The model under review builds one solid part; all positions refer to its coordinate system, in mm. A direction names the side the tool comes from. Round coordinates to 2 decimals unless told otherwise and drop trailing zeros. Loops run counter-clockwise (first coordinate to the right, second up) from the corner with the lowest first, then second, coordinate; pieces in that order, holes last. Notation, with made-up numbers: M 88.5,-32 L 116.5,-32 A8 cw 116.5,-24 Z; hole C 4,77.25 d3. An arc over 180 degrees is marked long. Return JSON: item names as keys, results as strings. Group by question number.
Q1. Draft analysis for pull direction Y (two halves, no side actions). For faces 5 (the face through (-47.94, 73.48, -0.18)), 6 (the face through (78.134, 0.474, 54.108)), 7 (the face through (89, -11, 44.45)), state which applies: pulls with the +Y half, pulls with the -Y half, needs draft (parallel to the pull), parting line crosses it, or undercut.
Q2. For faces 1 (the face through (63, 0, 57.15)), 2 (the face through (63, 0, 50.8)), 3 (the face through (49.2, -9.6, 52.6)), 4 (the face through (6, 6.35, 33)), list the 3-axis set-ups (+Z, -Z, +X, -X, +Y, -Y) from which the entire face can be reached by the end or side of a thin tool; tool diameter is ignored.
Q3. Consider section A-A (x = -31.75). Count the separate pieces of the cut face and the enclosed holes in it, and give its area (3 significant figures).
Q4. Clearance check with flat-ended pins moving along their axes: pin 1 Ø7 at (y, z) = (8.5, 27) entering from -X; pin 2 Ø24.5 at (x, z) = (52, 31.5) entering from -Y; pin 3 Ø16.5 at (x, y) = (31.75, 53.975) entering from -Z; pin 4 Ø8 at (x, y) = (22.5, -10.5) entering from +Z. State where each tip first meets the part, or that it passes through.
Q5. Consider section B-B (y = 39.5). State the section outline as (x, z) points.
Q6. To check wall thickness, follow line 1 along Y through (x, z) = (31, 7); line 2 along Y through (x, z) = (31.75, 6) (3 decimals); line 3 along Y through (x, z) = (88, 54). State the ranges of each line that lie inside material, in increasing order.
from build123d import *

# Parameters (mm, degrees)
F1_DEPTH = 76.2
F2_DEPTH = 12.7
F3_DEPTH = 6.35
F5_R     = 9.525
F6_R     = 10.7761659596
F7_DEPTH = 76.201
F8_R     = 6.35
F9_DEPTH = 12.7


with BuildPart() as f1:
    # F0 (on Front) → F1 (new body, symmetric)
    with BuildSketch(Plane.XZ):
        Polygon((-50.8, 12.7), (-50.8, -12.7), (50.8, -12.7), (50.8, 12.7), (44.45, 12.7), align=None)
    extrude(amount=F1_DEPTH, both=True)

    # F0 (on Front) → F2 (join, symmetric)
    with BuildSketch(Plane.XZ):
        with BuildLine():
            Line((44.45, 12.7), (50.8, 12.7))
            Line((50.8, 12.7), (50.8, 41.275))
            ThreePointArc((50.8, 41.275), (53.5898079092, 48.0101920908), (60.325, 50.8))
            Line((60.325, 50.8), (88.9, 50.8))
            Line((88.9, 50.8), (88.9, 57.15))
            Line((88.9, 57.15), (60.325, 57.15))
            ThreePointArc((60.325, 57.15), (49.0996798487, 52.5003201513), (44.45, 41.275))
            Line((44.45, 41.275), (44.45, 12.7))
        make_face()
    extrude(amount=F2_DEPTH, both=True)

    # F0 (on Front) → F3 (join, symmetric)
    with BuildSketch(Plane.XZ):
        with BuildLine():
            add(Edge.make_bspline(
                [(-50.8, 12.7), (-36.4359264535, 24.9142696717), (-6.0956798741, 63.0964294524), (39.4712934893, 57.15), (60.325, 57.15)],
                knots=[0, 0, 0, 0, 0.4989893673, 1, 1, 1, 1], degree=3))
            Line((-50.8, 12.7), (44.45, 12.7))
            Line((44.45, 12.7), (44.45, 41.275))
            ThreePointArc((44.45, 41.275), (49.0996798487, 52.5003201513), (60.325, 57.15))
        make_face()
    extrude(amount=F3_DEPTH, both=True)

    # F0 (on Front) → F4 (revolve)
    with BuildSketch(Plane.XZ):
        Polygon((88.9, 63.5), (88.9, 57.15), (88.9, 50.8), (88.9, 44.45), (114.3, 44.45), (114.3, 63.5), align=None)
    revolve(axis=Axis((88.9, 0, 53.975), (0, 0, 1)))

    # F5
    f5_edges = [f1.edges().sort_by_distance(p)[0] for p in [
        (50.8, -76.2, 0),
        (50.8, 76.2, 0),
        (-50.8, 76.2, 0),
        (-50.8, -76.2, 0),
    ]]
    fillet(f5_edges, radius=F5_R)

    # F6 (on face) → F7 (cut, through all)
    with BuildSketch(Plane.XY.offset(63.5)):
        with Locations((88.9, 0)):
            Circle(F6_R)
    extrude(amount=-F7_DEPTH, mode=Mode.SUBTRACT)

    # F8 (on Top) → F9 (cut, symmetric)
    with BuildSketch(Plane.XY):
        with Locations((-31.75, -53.975)):
            Circle(F8_R)
        with Locations((31.75, -53.975)):
            Circle(F8_R)
        with Locations((31.75, 53.975)):
            Circle(F8_R)
        with Locations((-31.75, 53.975)):
            Circle(F8_R)
    extrude(amount=F9_DEPTH, both=True, mode=Mode.SUBTRACT)


solid = f1.part
Values:
{
 "1": {"face 5": "pulls with the +Y half", "face 6": "undercut", "face 7": "needs draft"},
 "2": {"face 1": "+Z", "face 2": "-Z", "face 3": "+Z, -X, -Y", "face 4": "+Z, -X, +Y"},
 "3": {"separate pieces": "3", "enclosed holes": "0", "area": "3,450 mm2"},
 "4": {"pin 1": "stops at x = -38.42", "pin 2": "stops at y = -12.7", "pin 3": "stops at z = -12.7", "pin 4": "stops at z = 12.7"},
 "5": {"outline": "M -50.8,-12.7 L 50.8,-12.7 L 50.8,12.7 L -50.8,12.7 Z"},
 "6": {"line 1": "y = -76.2 to -60.28, -47.67 to 47.67, 60.28 to 76.2", "line 2": "y = -76.2 to -60.325, -47.625 to 47.625, 60.325 to 76.2", "line 3": "y = -25.38 to -10.74, 10.74 to 25.38"}
}
